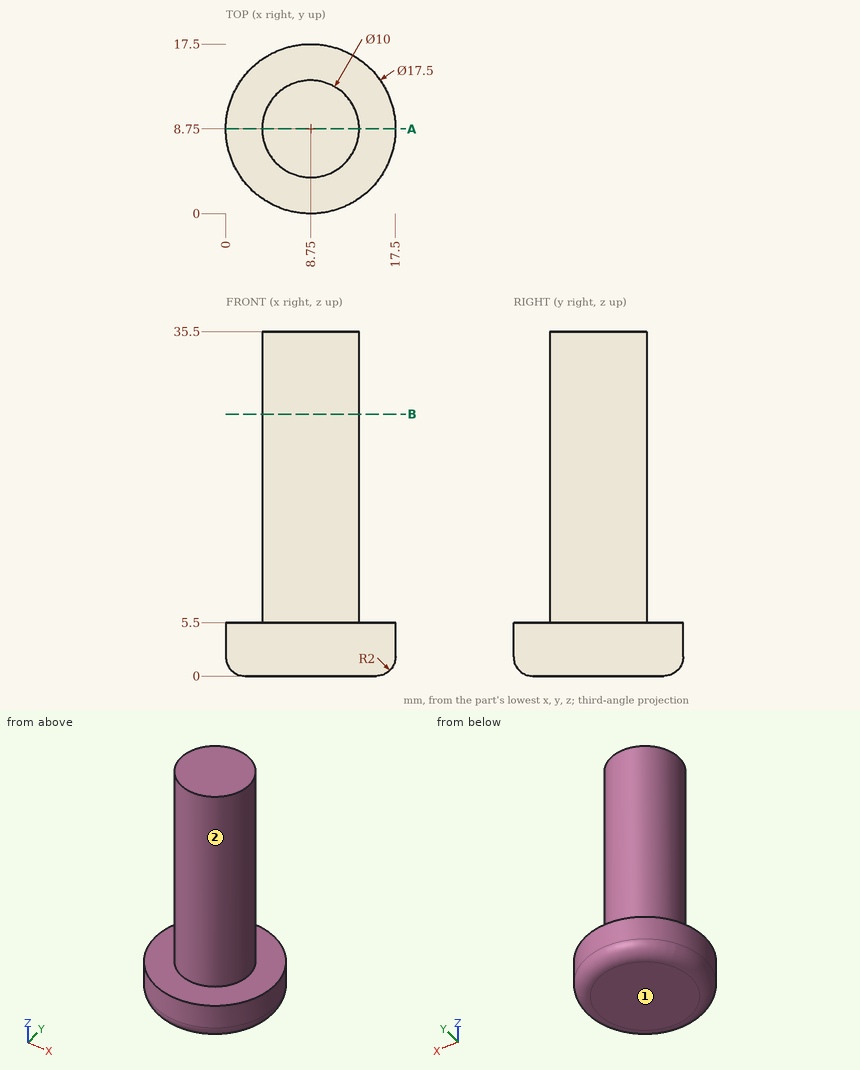
Verification items for this drawing (mm, ordinates from the low corner). A direction names the side the tool comes from. Coordinates: 2 decimals unless noted, no trailing zeros. Write each loop counter-clockwise with the first axis right and the second up, starting at its lowest first coordinate (ties: lowest second). Pieces come first, ordered by that corner, then holes. Notation, with made-up numbers: (-29.5, 52) -> (-13.5, 52) arc R10 ccw to (-13.5, 68) -> close; hole circle Ø2 at (84.25, 67.25). An arc over 180 degrees is marked (long way). Use CSV: the item, a comma, the result in double quotes. Start each with the question number.
Item 1: Cross-section at A-A, the plane y = 8.75. Record the cut outline in (x, z).
Item 2: Set-up check for the marked faces 1 and 2: record each of +Z, -Z, +X, -X, +Y, -Y from which the full face is reachable in a straight line by a thin tool's end or side.
Item 3: Depth check by flat-ended pin: pin 1 Ø5 at (x, z) = (4, 9) entering from +Y; pin 2 Ø2 at (y, z) = (4, 12) entering from -X; pin 3 Ø8 at (x, z) = (4, 21) entering from -Y. Enter the tip coordinate at first touch or a pass-through.
Item 4: Thickness scan on line 1 (Z direction, x = 3.5, y = 12.75); line 2 (Y direction, x = 9, z = 12); line 3 (Y direction, x = 5.5, z = 16). Record the ranges inside material, lowest first.
Item 5: Cross-section at B-B, the plane z = 27. Record the cut outline in (x, y).
Answers:
1,outline,"(0, 2) arc R2 ccw to (2, 0) -> (15.5, 0) arc R2 ccw to (17.5, 2) -> (17.5, 5.5) -> (13.75, 5.5) -> (13.75, 35.5) -> (3.75, 35.5) -> (3.75, 5.5) -> (0, 5.5) -> close"
2,face 1,"-Z, +X, -X, +Y, -Y"
2,face 2,"+Z"
3,pin 1,"y = 13.22"
3,pin 2,"x = 5.44"
3,pin 3,"y = 3.81"
4,line 1,"0 to 5.5"
4,line 2,"3.76 to 13.74"
4,line 3,"4.95 to 12.55"
5,outline,"circle Ø10 at (8.75, 8.75)"
